Geometry: final body of the model. Coordinates: model frame, mm. A direction names the side the tool comes from. Give positions to 0.01 mm unless a question says otherwise; leave off trailing zeros. Loops run counter-clockwise (first coordinate to the right, second up) from the corner with the lowest first, then second, coordinate; pieces in that order, holes last. Notation, with made-up numbers: M 35.25,-22.75 L 78.25,-22.75 A37 cw 78.25,14.25 Z; hole C 37.5,31 d3. An arc over 180 degrees is marked long. One line per question, with ' | ' between items. Start each with the question number.
from build123d import *

# Parameters (mm, degrees)
SKETCH1_R           = 7.45
BOSS_EXTRUDE1_DEPTH = 4.4
SKETCH2_R           = 2.95
CUT_EXTRUDE1_DEPTH  = 3.4
SKETCH3_OUTSIDE_W   = 24.262
SKETCH3_OUTSIDE_H   = 24.262
SKETCH3_OUTSIDE_R   = 6.3
CUT_EXTRUDE2_DEPTH  = 5
CUT_EXTRUDE2_DRAFT  = -17
SHELL1_2_OUTLINE_W  = 4.15
SHELL1_2_OUTLINE_H  = 0.2
CUT_EXTRUDE3_START  = -3.4
SKETCH4_R           = 4.15
SKETCH4_R_2         = 3.95
CUT_EXTRUDE3_DEPTH  = 3.4
SKETCH5_R           = 2.9
BOSS_EXTRUDE2_DEPTH = 3
SKETCH6_R           = 1.7
CUT_EXTRUDE4_DEPTH  = 3.3


# Read off the part's stored shape, not the designer's step: Shell1
with BuildPart() as part:
    # Sketch1 → Boss-Extrude1 (new body)
    with BuildSketch(Plane(origin=(0, 0, 0), x_dir=(1, 0, 0), z_dir=(0, 1, 0))):
        with Locations(Location((0, 0, 0), (0, 0, 270))):
            Circle(SKETCH1_R)
    extrude(amount=BOSS_EXTRUDE1_DEPTH)

    # Sketch2 → Cut-Extrude1 (cut)
    with BuildSketch(Plane.XZ):
        with Locations(Location((0, 0, 0), (0, 0, 270))):
            Circle(SKETCH2_R)
    extrude(amount=-CUT_EXTRUDE1_DEPTH, mode=Mode.SUBTRACT)


with BuildPart() as cut_extrude2_tool:
    # Sketch3 outside → Cut-Extrude2 (with draft: the straight prism first)
    with BuildSketch(Plane(origin=(0, 0, 0), x_dir=(-1, 0, 0), z_dir=(0, -1, 0))):
        Rectangle(SKETCH3_OUTSIDE_W, SKETCH3_OUTSIDE_H)
        Circle(SKETCH3_OUTSIDE_R, mode=Mode.SUBTRACT)
    extrude(amount=-CUT_EXTRUDE2_DEPTH)
    # Cut-Extrude2: the draft: its side faces are tilted about the plane it starts from
    cut_extrude2_sides = [cut_extrude2_tool.faces().sort_by_distance(p)[0] for p in [
        (0, 2.5, 12.131),
        (-12.131, 2.5, 0),
        (0, 2.5, -12.131),
        (12.131, 2.5, 0),
        (6.3, 2.5, 0),
    ]]
    draft(cut_extrude2_sides, Plane(origin=(0, 0, 0), x_dir=(-1, 0, 0), z_dir=(0, -1, 0)), CUT_EXTRUDE2_DRAFT)


with BuildPart() as part_1:
    add(part.part)

    # Cut-Extrude2: cut by cut_extrude2_tool
    add(cut_extrude2_tool.part, mode=Mode.SUBTRACT)

    # Shell1 outline → Shell1 (revolve, cut)
    with BuildSketch(Plane.XY):
        Polygon((4.15, 4.4), (4.15, 1.2), (5.41204671, 1.2), (6.25, 3.940821713), (6.25, 4.4), align=None)
    revolve(axis=Axis((0, 0, 0), (0, 1, 0)), mode=Mode.SUBTRACT)

    # Shell1 2 outline → Shell1 2 (revolve)
    with BuildSketch(Plane.XY):
        with Locations((2.075, 4.5)):
            Rectangle(SHELL1_2_OUTLINE_W, SHELL1_2_OUTLINE_H)
    revolve(axis=Axis((0, 0, 0), (0, 1, 0)))

    # Sketch4 → Cut-Extrude3 (cut)
    with BuildSketch(Plane(origin=(0, 4.6, 0), x_dir=(1, 0, 0), z_dir=(0, 1, 0)).offset(CUT_EXTRUDE3_START)):
        Circle(SKETCH4_R)
        with Locations(Location((0, 0, 0), (0, 0, 270))):
            Circle(SKETCH4_R_2, mode=Mode.SUBTRACT)
    extrude(amount=CUT_EXTRUDE3_DEPTH, mode=Mode.SUBTRACT)

    # Sketch5 → Boss-Extrude2 (add)
    with BuildSketch(Plane(origin=(0, 4.6, 0), x_dir=(1, 0, 0), z_dir=(0, 1, 0))):
        with Locations(Location((0, 0, 0), (0, 0, 270))):
            Circle(SKETCH5_R)
    extrude(amount=BOSS_EXTRUDE2_DEPTH)

    # Sketch6 → Cut-Extrude4 (cut)
    with BuildSketch(Plane(origin=(0, 7.6, 0), x_dir=(1, 0, 0), z_dir=(0, 1, 0))):
        with Locations(Location((0, 0, 0), (0, 0, 270))):
            Circle(SKETCH6_R)
    extrude(amount=-CUT_EXTRUDE4_DEPTH, mode=Mode.SUBTRACT)


solid = part_1.part
Q1. Material intervals for L1, parallel to X at y = 4.25, z = 0; L2, parallel to X at y = 2, z = -0.25; L3, parallel to Y at x = 4, z = 0.75, sorted ascending.
Q2. Section D-D, the plane y = 0.5. Output: boundary loops of the cut face in (x, z).
Q3. Section C-C, the plane y = 1.5. Output: boundary loops of the cut face in (x, z).
Q4. Section B-B, the plane x = 0. Output: boundary loops of the cut face in (y, z), plus the area to 3 significant figures.
Q5. Draft query along Z for faces 1 (the flat face through (0, 3.4, 0)), 2 (the conical face through (-1.185, 1.371, 5.335)), 3 (the cylindrical face through (-6.61, 4.08, 3.44)), 4 (the flat face through (-1, 0, 3)). Return one class per face: released by +Z, released by -Z, zero draft, split by the parting line, or undercut.
Q6. Contact query for flat-ended pins moving along their axis: pin 1 (2 mm diameter, centred on x = 5.5, y = 3, fed in from -Z); pin 2 (1.5 mm diameter, centred on x = 5, y = 2.5, fed in from +Z); pin 3 (1.7 mm diameter, centred on x = 0.5, z = 0.5, fed in from +Y); pin 4 (8.5 mm diameter, centred on x = 1.5, z = 0, fed in from +Y). Output: stop coordinate, or through.
Q7. Section A-A, the plane z = 0. Output: boundary loops of the cut face in (x, y), plus the area to 3 significant figures.
Q8. Set-up query: faces 5 (the flat face through (4, 1.2, 2)), 6 (the flat face through (-2, 7.6, 0)), 7 (the cylindrical face through (-2.88, 1.68, 0.64)). Return all of +Z, -Z, +X, -X, +Y, -Y with unobstructed straight access to the full face (end or side cutting, diameter ignored); none if empty.
Model answer:
1) L1: x = -7.45 to -6.25, -3.95 to 3.95, 6.25 to 7.45 | L2: x = -6.91 to -5.65, -3.94 to -2.94, 2.94 to 3.94, 5.65 to 6.91 | L3: y = 0 to 1.2
2) outline: C 0,0 d12.91; hole C 0,0 d5.9
3) outline: C 0,0 d13.52; C 0,0 d7.9; hole C 0,0 d11.01; hole C 0,0 d5.9
4) outline: M 0,-6.3 L 3.76,-7.45 L 4.4,-7.45 L 4.4,-6.25 L 3.94,-6.25 L 1.2,-5.41 L 1.2,-3.95 L 4.6,-3.95 L 4.6,-2.9 L 7.6,-2.9 L 7.6,-1.7 L 4.3,-1.7 L 4.3,1.7 L 7.6,1.7 L 7.6,2.9 L 4.6,2.9 L 4.6,3.95 L 1.2,3.95 L 1.2,5.41 L 3.94,6.25 L 4.4,6.25 L 4.4,7.45 L 3.76,7.45 L 0,6.3 L 0,2.95 L 3.4,2.95 L 3.4,-2.95 L 0,-2.95 Z | area: 36.5 mm^2
5) face 1: undercut | face 2: undercut | face 3: split by the parting line | face 4: zero draft
6) pin 1: stops at z = -5.73 | pin 2: stops at z = 5.71 | pin 3: stops at y = 4.3 | pin 4: stops at y = 7.6
7) outline: M -7.45,3.76 L -6.3,0 L -2.95,0 L -2.95,3.4 L 2.95,3.4 L 2.95,0 L 6.3,0 L 7.45,3.76 L 7.45,4.4 L 6.25,4.4 L 6.25,3.94 L 5.41,1.2 L 3.95,1.2 L 3.95,4.6 L 2.9,4.6 L 2.9,7.6 L 1.7,7.6 L 1.7,4.3 L -1.7,4.3 L -1.7,7.6 L -2.9,7.6 L -2.9,4.6 L -3.95,4.6 L -3.95,1.2 L -5.41,1.2 L -6.25,3.94 L -6.25,4.4 L -7.45,4.4 Z | area: 36.5 mm^2
8) face 5: +Y | face 6: +Z, -Z, +X, -X, +Y | face 7: -Y
